Check sheet for the modelled part. Datum: model origin and axes. Units: mm. A direction names the side the tool comes from. Give positions to 0.01 mm unless a question says otherwise; leave off trailing zeros. Order: outer loops, then holes, each group sorted by start corner. A loop starts at its lowest first (then second) coordinate and runs counter-clockwise, first axis right, second up. Notation, with made-up numbers: (-40, 89.25) - (-32, 89.25) arc R29 cw to (-32, 124.25) - close; hole circle Ø4 at (7.5, -13.5). An arc over 180 degrees is marked (long way). Answer in a Markdown table with one row per item.
from build123d import *

# Parameters (mm, degrees)
SKETCH1_R           = 5.25
SKETCH1_R_2         = 3
BOSS_EXTRUDE1_DEPTH = 12
SKETCH2_R           = 4
SKETCH2_R_2         = 1.5
BOSS_EXTRUDE2_DEPTH = 8
CUT_EXTRUDE2_START  = -8
CUT_EXTRUDE2_DEPTH  = 8


with BuildPart() as part:
    # Sketch1 → Boss-Extrude1 (new body)
    with BuildSketch(Plane(origin=(0, 0, 0), x_dir=(1, 0, 0), z_dir=(0, 1, 0))):
        with Locations(Location((0, 0, 0), (0, 0, 270))):
            Circle(SKETCH1_R)
        with Locations(Location((0, 0, 0), (0, 0, 270))):
            Circle(SKETCH1_R_2, mode=Mode.SUBTRACT)
    extrude(amount=BOSS_EXTRUDE1_DEPTH)

    # Sketch2 → Boss-Extrude2 (add)
    with BuildSketch(Plane(origin=(0, 12, 0), x_dir=(1, 0, 0), z_dir=(0, 1, 0))):
        with Locations(Location((0, 0, 0), (0, 0, 270))):
            Circle(SKETCH2_R)
        with Locations(Location((0, 0, 0), (0, 0, 270))):
            Circle(SKETCH2_R_2, mode=Mode.SUBTRACT)
    extrude(amount=BOSS_EXTRUDE2_DEPTH)

    # Sketch4 → Cut-Extrude2 (cut)
    with BuildSketch(Plane(origin=(0, 20, 0), x_dir=(1, 0, 0), z_dir=(0, 1, 0)).offset(CUT_EXTRUDE2_START)):
        with BuildLine():
            Line((-1.936491673, 3.5), (1.936491673, 3.5))
            ThreePointArc((1.936491673, 3.5), (0, 4), (-1.936491673, 3.5))
        make_face()
    extrude(amount=CUT_EXTRUDE2_DEPTH, mode=Mode.SUBTRACT)


solid = part.part
(1) Mould release check, pull along Z, two halves, no side actions. Record for faces 4 (the flat face through (0, 20, 2)), 5 (the flat face through (0, 16, -3.5)), 6 (the flat face through (-1.3, 12, 1.3)): pulls with the +Z half, pulls with the -Z half, needs draft (parallel to the pull), parting line crosses it, or undercut.
Geometry says:
| item | result |
|---|---|
| face 4 | needs draft |
| face 5 | pulls with the -Z half |
| face 6 | undercut |
(2) Cross-section at B-B, the plane x = 0. Record the cut outline in (y, z).
Geometry says:
| item | result |
|---|---|
| outline | (0, -5.25) - (12, -5.25) - (12, -3.5) - (20, -3.5) - (20, -1.5) - (12, -1.5) - (12, -3) - (0, -3) - close; (0, 3) - (12, 3) - (12, 1.5) - (20, 1.5) - (20, 4) - (12, 4) - (12, 5.25) - (0, 5.25) - close |
(3) Access from +Z, -Z, +X, -X, +Y, -Y to the whole of each face (thin tool, end or side, straight path). Record for faces 1 (the cylindrical face through (0.45, 15.94, 1.43)), 2 (the cylindrical face through (0.9, 5.92, 2.86)), 3 (the flat face through (0, 12, -4)).
Geometry says:
| item | result |
|---|---|
| face 1 | +Y, -Y |
| face 2 | -Y |
| face 3 | +Y |
(4) Cross-section at C-C, the plane y = 18. Record the cut outline in (x, z), then the cut area to 3 significant figures.
Geometry says:
| item | result |
|---|---|
| outline | (-1.94, -3.5) - (1.94, -3.5) arc R4 ccw (long way) to start; hole circle Ø3 at (0, 0) |
| area | 41.9 mm² |
(5) Thickness scan on L1, parallel to X at y = 14.75, z = 0; L2, parallel to X at y = 7.75, z = -0.5; L3, parallel to Y at x = 4.5, z = -2.5. Record the ranges inside material, lowest first.
Geometry says:
| item | result |
|---|---|
| L1 | -4 to -1.5, 1.5 to 4 |
| L2 | -5.23 to -2.96, 2.96 to 5.23 |
| L3 | 0 to 12 |
(6) Gauge pin test, flat ends, axial feed: P1, Ø5, axis at x = 0, z = 0, coming from the -Y side; P2, Ø2, axis at y = 12, z = 1.5, coming from the -X side; P3, Ø1, axis at x = 2, y = 17.5, coming from the -Z side. Record the tip position at first contact, or that the pin passes through.
Geometry says:
| item | result |
|---|---|
| P1 | y = 12 |
| P2 | x = -5.23 |
| P3 | z = -3.5 |
(7) Cross-section at D-D, the plane x = 3.5. Record the cut outline in (y, z), then the cut area to 3 significant figures.
Geometry says:
| item | result |
|---|---|
| outline | (0, -3.91) - (12, -3.91) - (12, -1.94) - (20, -1.94) - (20, 1.94) - (12, 1.94) - (12, 3.91) - (0, 3.91) - close |
| area | 125 mm² |
(8) Cross-section at A-A, the plane z = 0. Record the cut outline in (x, y).
Geometry says:
| item | result |
|---|---|
| outline | (-5.25, 0) - (-3, 0) - (-3, 12) - (-1.5, 12) - (-1.5, 20) - (-4, 20) - (-4, 12) - (-5.25, 12) - close; (1.5, 12) - (3, 12) - (3, 0) - (5.25, 0) - (5.25, 12) - (4, 12) - (4, 20) - (1.5, 20) - close |
